Part model, mm, in its own coordinate system. A direction names the side the tool comes from. Give positions to 0.01 mm unless a question says otherwise; leave off trailing zeros. Order: outer loops, then holes, each group sorted by start corner. A loop starts at its lowest first (then second) coordinate and runs counter-clockwise, first axis right, second up. Notation, with made-up numbers: (31.5, -25.5) - (65.5, -25.5) arc R20 cw to (65.5, -16.5) - close; hole circle Ø1 at (24, 79). An arc over 180 degrees is marked (long way). One line per item, written item: value.
Autodesk Inventor part; units mm, degrees
ref_plane "ANBAU_XY" through (0, 0, 0) normal (-1, 0, 0) x (0, 0, -1)
ref_plane "ANBAU_YZ" through (0, 0, 0) normal (0, 0, -1) x (0, -1, 0)
ref_plane "ANBAU_ZX" through (0, 0, 0) normal (0, -1, 0) x (-1, 0, 0)
sketch "Sketch_1" plane through (0, 0, 0) normal (0, 0, 1) x (1, 0, 0)
  line L0 (8, 0) -> (-3, 0)
  line L1 (-3, 0) -> (-3, 2.75)
  line L2 (-3, 2.75) -> (0, 2.75)
  line L3 (0, 2.75) -> (0, 1.8)
  line L4 (0, 1.8) -> (0.51, 1.5)
  line L5 (0.51, 1.5) -> (7.6935, 1.5)
  line L6 (7.6935, 1.5) -> (8, 1.1935)
  line L7 (8, 1.1935) -> (8, 0)
  line L8 (8, 0) -> (-3, 0)
revolve "Revolution1" add sketch "Sketch_1" angle 360 about axis through (8, 0, 0) along (1, 0, 0)
thread "Thread1"
sketch "Sketch_6" plane through (0, 0, 0) normal (0, 0, 1) x (1, 0, 0)
  line L0 (0, 0) -> (-3, 0)
  line L1 (-3, 3.3) -> (-3, 2.45)
  line L2 (-3, 2.45) -> (-2.7, 2.75)
  line L3 (-2.7, 2.75) -> (-0.215, 2.75)
  line L4 (-0.215, 2.75) -> (0, 2.535)
  line L5 (0, 2.535) -> (0, 3.3)
  line L6 (0, 3.3) -> (-3, 3.3)
revolve "Revolution2" cut sketch "Sketch_6" angle 360 about axis through (0, 0, 0) along (1, 0, 0)
sketch "Sketch3" plane through (-3, 0, 0) normal (-1, 0, 0) x (0, 0, 1)
  point P0 (0, 0)
hole "Hole1" at (-3, 0, 0) direction (1, 0, 0) diameter 2.5 depth 1.3 tip angle 120 countersink diameter 2.85 countersink angle 90
sketch "Sketch_2" plane through (-3, 0, 0) normal (1, 0, 0) x (0, 0, -1)
  line L0 (-1.25, -0.7217) -> (0, -1.4434)
  line L1 (0, -1.4434) -> (1.25, -0.7217)
  line L2 (1.25, -0.7217) -> (1.25, 0.7217)
  line L3 (1.25, 0.7217) -> (0, 1.4434)
  line L4 (0, 1.4434) -> (-1.25, 0.7217)
  line L5 (-1.25, 0.7217) -> (-1.25, -0.7217)
extrude "Extrusion1" cut sketch "Sketch_2" along normal mid plane 2.6
ref_plane "ANBAU_XY" through (0, 0, 0) normal (-1, 0, 0) x (0, 0, -1)
ref_plane "ANBAU_YZ" through (0, 0, 0) normal (0, 0, -1) x (0, -1, 0)
ref_plane "ANBAU_ZX" through (0, 0, 0) normal (0, -1, 0) x (-1, 0, 0)
ref_plane "IP1_XY" through (0, 0, 0) normal (1, 0, 0) x (0, 0, -1)
ref_plane "IP1_YZ" through (0, 0, 0) normal (0, 0, -1) x (0, 1, 0)
ref_plane "IP1_ZX" through (0, 0, 0) normal (0, 1, 0) x (1, 0, 0)
ref_plane "IP2_XY" through (-3, 0, 0) normal (1, 0, 0) x (0, 0, -1)
ref_plane "IP2_YZ" through (-3, 0, 0) normal (0, 0, -1) x (0, 1, 0)
ref_plane "IP2_ZX" through (-3, 0, 0) normal (0, 1, 0) x (1, 0, 0)
ref_plane "IP3_XY" through (8, 0, 0) normal (1, 0, 0) x (0, 0, -1)
ref_plane "IP3_YZ" through (8, 0, 0) normal (0, 0, -1) x (0, 1, 0)
ref_plane "IP3_ZX" through (8, 0, 0) normal (0, 1, 0) x (1, 0, 0)
properties part number "ISO-4762 M3x8"
1) Slice it at A-A on x = 1.5. Write the cut outline in (y, z).
Answer:
outline: circle Ø3 at (0, 0)
2) Which spindle directions (+Z, -Z, +X, -X, +Y, -Y) get a long thin tool onto all of the face, cutting with end or side? Do faces 4 (the face through (0, -2, -1)), 5 (the face through (-1.44, -0.596, -2.685)), 6 (the face through (-2.359, 1.088, 0.616)). Say none if no direction does.
Answer:
face 4: +X
face 5: +X, -X
face 6: -X
3) Drop flat-ended pins along their axis: P1, Ø1.4, axis at x = -2.5, y = 0.5, coming from the -Z side; P2, Ø3, axis at x = -1.5, y = -2, coming from the +Z side; P3, Ø0.7, axis at y = 1, z = 0, coming from the -X side; P4, Ø2, axis at x = 3.5, z = 1, coming from the -Y side. Give the stop position or say it passes through.
Answer:
P1: stops at z = -2.75
P2: stops at z = 2.7
P3: stops at x = -1.7
P4: stops at y = -1.5
4) Wall check: line 1 along X through (y, z) = (1.9, -1.2); line 2 along Z through (x, y) = (4.5, -0.4); line 3 along Z through (x, y) = (0.75, -0.25). Give the ranges that are in metal, low to high. Write a range as [from, to].
Answer:
line 1: x = [-3, 0]
line 2: z = [-1.45, 1.45]
line 3: z = [-1.48, 1.48]
5) Two-plate mould, pull along Z, no slides. Class faces 1 (the face through (4.15, -1.5, 0.07)), 2 (the face through (-2.359, -1.088, -0.616)), 3 (the face through (-3, 0, -2)): pulls with the +Z half, pulls with the -Z half, needs draft (parallel to the pull), parting line crosses it, or undercut.
Answer:
face 1: parting line crosses it
face 2: undercut
face 3: needs draft
6) Slice it at B-B on x = 0.25. Write the cut outline in (y, z).
Answer:
outline: circle Ø3.31 at (0, 0)
